Here's how the part is built. I have some questions about the finished solid (model axes, mm). Coordinates: 2 decimals unless noted, no trailing zeros. Order: outer loops, then holes, each group sorted by start corner. A loop starts at its lowest first (then second) coordinate and runs counter-clockwise, first axis right, second up. Notation, with made-up numbers: (-26, -28) - (-7, -28) arc R18 cw to (-7, -10) - close; hole circle Ø2 at (-1.5, 12). An arc over 180 degrees is marked (long way). Answer in a Markdown table with one row per item. Add a question column.
Item 1: If I drill on line 1 along Z through (x, y) = (-95, 0.6); line 2 along Z through (x, y) = (126.5, 2.65); line 3 along X through (y, z) = (0.9, 82.5), over which ranges is the centre line in solid material (lowest first)? Write a range as from..to.
Item 2: I want a section at A-A (y = 0.8). Please give me the cut outline in (x, z).
Item 3: I want a section at B-B (z = 45.5). Please give me the cut outline in (x, y), plus the area to 3 significant figures.
Item 4: I want a section at C-C (x = -112). Please give me the cut outline in (y, z).
Item 5: Will this pin go through, and if not, where does the flat tip stop? pin 1 Ø10 at (x, z) = (-1, -161) entering from -Y.
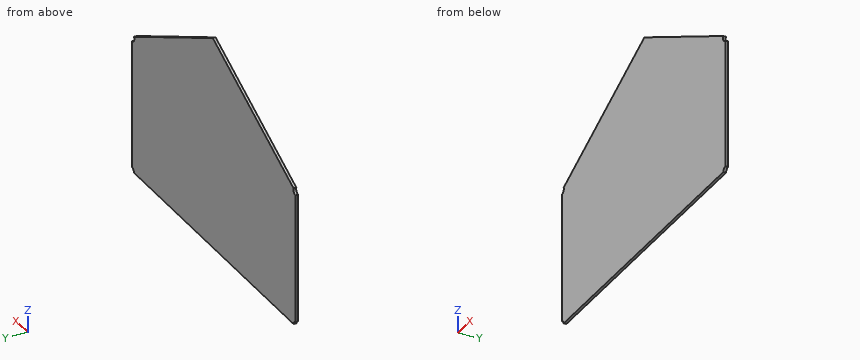
```python
from build123d import *

# Parameters (mm, degrees)
BOSS_EXTRUDE1_DEPTH = 4
SKETCH3_R           = 5.470416759
SKETCH3_R_2         = 5.136398205
SKETCH3_R_3         = 5.743645838
SKETCH3_R_4         = 6.779267961
CUT_EXTRUDE2_DEPTH  = 85


with BuildPart() as part:
    # Sketch1 → Boss-Extrude1 (new body)
    with BuildSketch(Plane(origin=(0, 0, 0), x_dir=(1, 0, 0), z_dir=(0, 1, 0))):
        with BuildLine():
            Line((-234.498829852, -2.772290193), (-7.346998412, -115.1588183))
            Line((-7.346998412, -115.1588183), (215.490107836, -2.772308919))
            ThreePointArc((215.490107836, -2.772308919), (215.494120314, -2.768622763), (215.495604699, -2.763380215))
            Line((215.495604699, -2.763380215), (215.495604699, 197.217709807))
            ThreePointArc((215.495604699, 197.217709807), (215.492675767, 197.224780875), (215.485604699, 197.227709807))
            Line((215.485604699, 197.227709807), (-234.494395301, 197.227709807))
            ThreePointArc((-234.494395301, 197.227709807), (-234.501466368, 197.224780875), (-234.504395301, 197.217709807))
            Line((-234.504395301, 197.217709807), (-234.504395301, -2.763327228))
            ThreePointArc((-234.504395301, -2.763327228), (-234.502890756, -2.768602381), (-234.498829852, -2.772290193))
        make_face()
    extrude(amount=BOSS_EXTRUDE1_DEPTH)

    # Sketch3 → Cut-Extrude2 (cut)
    with BuildSketch(Plane(origin=(0, 4, 0), x_dir=(1, 0, 0), z_dir=(0, 1, 0))):
        with Locations((-234.494395301, -2.763327228)):
            Circle(SKETCH3_R)
        with Locations((-234.494395301, 197.217709807)):
            Circle(SKETCH3_R_2)
        with Locations((215.485604699, 197.217709807)):
            Circle(SKETCH3_R_3)
        with Locations((215.485604699, -2.763380215)):
            Circle(SKETCH3_R_4)
    extrude(amount=-CUT_EXTRUDE2_DEPTH, mode=Mode.SUBTRACT)


solid = part.part
```
Values follow:
| question | item | result |
|---|---|---|
| 1 | line 1 | z = -197.23..71.79 |
| 1 | line 2 | z = -197.23..47.65 |
| 1 | line 3 | x = -73.36..57.41 |
| 2 | outline | (-234.5, -192.08) arc R5.14 cw to (-229.36, -197.23) - (209.74, -197.23) arc R5.74 cw to (215.5, -191.47) - (215.5, -4.02) arc R6.78 cw to (209.44, 5.83) - (-7.35, 115.16) - (-229.6, 5.2) arc R5.47 cw to (-234.5, -2.71) - close |
| 3 | outline | (-148.14, 0) - (130.77, 0) - (130.77, 4) - (-148.14, 4) - close |
| 3 | area | 1,120 mm^2 |
| 4 | outline | (0, -197.23) - (4, -197.23) - (4, 63.38) - (0, 63.38) - close |
| 5 | pin 1 | stops at y = 0 |
